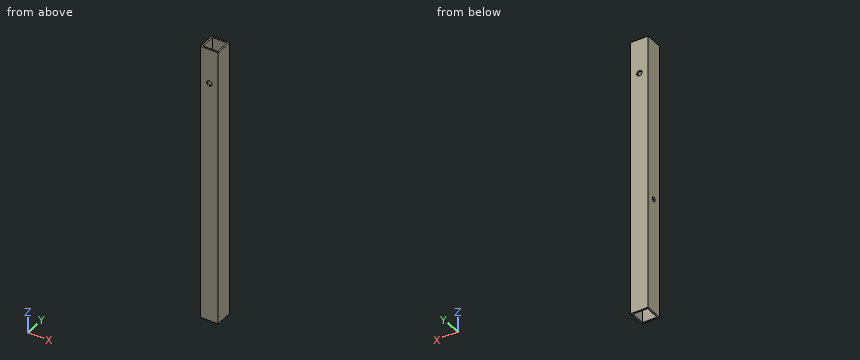
```python
from build123d import *

# Parameters (mm, degrees)
SKETCH1_W                   = 19.05
SKETCH1_H                   = 19.05
SKETCH1_W_2                 = 15.875
SKETCH1_H_2                 = 15.875
BOSS_EXTRUDE1_DEPTH         = 152.4
SKETCH2_R                   = 2.8956
BASEPLATE_MOUNT_HOLE_DEPTH  = 154.881084364
PS_BRACKET_MOUNT_HOLE_REACH = 155.881
SKETCH3_R                   = 2.4257


with BuildPart() as part:
    # Sketch1 → Boss-Extrude1 (new, symmetric)
    with BuildSketch(Plane(origin=(0, 0, 0), x_dir=(0, -1, 0), z_dir=(0, 0, 1))):
        Rectangle(SKETCH1_W, SKETCH1_H)
        Rectangle(SKETCH1_W_2, SKETCH1_H_2, mode=Mode.SUBTRACT)
    extrude(amount=BOSS_EXTRUDE1_DEPTH, both=True)

    # Sketch2 → Baseplate Mount Hole (cut, through all)
    with BuildSketch(Plane(origin=(0, 9.525, 0), x_dir=(1, 0, 0), z_dir=(0, 1, 0))):
        with Locations(Location((0, -114.3, 0), (0, 0, 180))):
            Circle(SKETCH2_R)
    extrude(amount=-BASEPLATE_MOUNT_HOLE_DEPTH, mode=Mode.SUBTRACT)

    # Sketch3 → PS Bracket Mount Hole (cut, up to next)
    with BuildSketch(Plane.ZY.offset(9.525), mode=Mode.PRIVATE) as ps_bracket_mount_hole_sk1:
        with Locations((-25.4, 0)):
            Circle(SKETCH3_R)
    ps_bracket_mount_hole_tool1 = extrude(ps_bracket_mount_hole_sk1.sketch, amount=-PS_BRACKET_MOUNT_HOLE_REACH, mode=Mode.PRIVATE) & part.part
    add(ps_bracket_mount_hole_tool1.solids().sort_by_distance((-9.525, 0, -25.4))[0], mode=Mode.SUBTRACT)


solid = part.part
```
The listing builds one solid part. Answer for the finished solid, in the listing's coordinates (mm). Coordinates: 2 decimals unless noted, no trailing zeros. Write each loop counter-clockwise with the first axis right and the second up, starting at its lowest first coordinate (ties: lowest second). Pieces come first, ordered by that corner, then holes. Notation, with made-up numbers: (-2.75, 4) - (15.25, 4) arc R23 cw to (15.25, 43) - close; hole circle Ø3 at (28.5, 65). An arc over 180 degrees is marked (long way). One line per item, written item: value.
1) Find section C-C (z = 114.3). Give the vertices of the cut face in (x, y) (1 decimal).
Geometry check:
outline: (-9.5, -9.5) - (-2.9, -9.5) - (-2.9, -7.9) - (-7.9, -7.9) - (-7.9, 7.9) - (-2.9, 7.9) - (-2.9, 9.5) - (-9.5, 9.5) - close; (2.9, -9.5) - (9.5, -9.5) - (9.5, 9.5) - (2.9, 9.5) - (2.9, 7.9) - (7.9, 7.9) - (7.9, -7.9) - (2.9, -7.9) - close
2) Find section B-B (z = -130.5). Give the vertices of the cut face in (x, y) (1 decimal), and give its area (3 significant figures).
Geometry check:
outline: (-9.5, -9.5) - (9.5, -9.5) - (9.5, 9.5) - (-9.5, 9.5) - close; hole (-7.9, -7.9) - (7.9, -7.9) - (7.9, 7.9) - (-7.9, 7.9) - close
area: 111 mm2
3) Consider line 1 along X through (y, z) = (-6.75, -18) (1 decimal); line 2 along Z through (x, y) = (0.25, -8.25). Determine where each line is inside the solid, lowest interval first. Write a range as from..to.
Geometry check:
line 1: x = -9.5..-7.9, 7.9..9.5
line 2: z = -152.4..111.42, 117.18..152.4
4) This flat-tipped pin is pushed along its axis until it touches: pin 1 Ø5 at (x, z) = (0, 114.3) entering from -Y. Where does it stop, or does it pass through?
Geometry check:
pin 1: passes through
5) Find section A-A (x = 0). Give the vertices of the cut face in (y, z) (1 decimal), and give its area (3 significant figures).
Geometry check:
outline: (-9.5, -152.4) - (-7.9, -152.4) - (-7.9, 111.4) - (-9.5, 111.4) - close; (-9.5, 117.2) - (-7.9, 117.2) - (-7.9, 152.4) - (-9.5, 152.4) - close; (7.9, -152.4) - (9.5, -152.4) - (9.5, 111.4) - (7.9, 111.4) - close; (7.9, 117.2) - (9.5, 117.2) - (9.5, 152.4) - (7.9, 152.4) - close
area: 949 mm2
